from build123d import *

# Parameters (mm, degrees)
F0_W     = 50
F0_H     = 50
F1_DEPTH = 6
F3_D     = 5
F5_D     = 25


with BuildPart() as f1:
    # F0 (on Top) → F1 (new body)
    with BuildSketch(Plane.XY):
        Rectangle(F0_W, F0_H)
    extrude(amount=F1_DEPTH)

    # F3 (through all)
    with Locations(Plane.XY.offset(6)):
        with Locations((0, 18), (18, 0), (0, -18), (-18, 0)):
            Hole(F3_D / 2)

    # F5 (through all)
    with Locations(Plane.XY.offset(6)):
        with Locations((0, 0)):
            Hole(F5_D / 2)


solid = f1.part
Model file for the job. Use its own axes, mm. Give positions to 0.01 mm unless a question says otherwise; leave off trailing zeros. Order: outer loops, then holes, each group sorted by start corner. A loop starts at its lowest first (then second) coordinate and runs counter-clockwise, first axis right, second up. Notation, with made-up numbers: (-20, -24.75) -> (23, -24.75) arc R16 cw to (23, -13.75) -> close; hole circle Ø3 at (54.5, -27). An arc over 180 degrees is marked (long way). Use CSV: the item, a comma, the result in double quotes.
1. Drill centre lines: line 1 along Y through (x, z) = (0, 4.15); line 2 along Y through (x, z) = (-18, 4.55); line 3 along X through (y, z) = (-1, 3.1). Where is each one in solid material? Low to high. Write a range as from..to.
Outcome:
line 1,"-25..-20.5, -15.5..-12.5, 12.5..15.5, 20.5..25"
line 2,"-25..-2.5, 2.5..25"
line 3,"-25..-20.29, -15.71..-12.46, 12.46..15.71, 20.29..25"
2. Band-saw the part on C-C, the plane z = 3.1. Give the cut face in (x, y).
Outcome:
outline,"(-25, -25) -> (25, -25) -> (25, 25) -> (-25, 25) -> close; hole circle Ø5 at (-18, 0); hole circle Ø25 at (0, 0); hole circle Ø5 at (0, -18); hole circle Ø5 at (0, 18); hole circle Ø5 at (18, 0)"
3. Drop a flat-ended pin along its axis: pin 1 (4 mm diameter, centred on x = 0, y = 18, fed in from -Z). Give the stop position or say it passes through.
Outcome:
pin 1,"through"
4. Mould opens along Y. For faces 1 (the flat face through (-5.9, 11.5, 6)), 2 (the flat face through (0, -25, 3)), 3 (the cylindrical face through (-15.5, 0.1, 3)) say: +Y half, -Y half, draft (parallel to the pull), parting line (faces both ways), or undercut.
Outcome:
face 1,"draft"
face 2,"-Y half"
face 3,"undercut"
5. Band-saw the part on A-A, the plane x = 18. Give the cut face in (y, z), then the cut area to 3 significant figures.
Outcome:
outline,"(-25, 0) -> (-2.5, 0) -> (-2.5, 6) -> (-25, 6) -> close; (2.5, 0) -> (25, 0) -> (25, 6) -> (2.5, 6) -> close"
area,"270 mm²"
6. Band-saw the part on B-B, the plane y = 0. Give the cut face in (x, z).
Outcome:
outline,"(-25, 0) -> (-20.5, 0) -> (-20.5, 6) -> (-25, 6) -> close; (-15.5, 0) -> (-12.5, 0) -> (-12.5, 6) -> (-15.5, 6) -> close; (12.5, 0) -> (15.5, 0) -> (15.5, 6) -> (12.5, 6) -> close; (20.5, 0) -> (25, 0) -> (25, 6) -> (20.5, 6) -> close"
